Part model, mm, in its own coordinate system. A direction names the side the tool comes from. Round coordinates to 2 decimals unless told otherwise and drop trailing zeros.
from build123d import *

# Parameters (mm, degrees)
SKETCH1_W            = 144.702517086
SKETCH1_H            = 104.868678114
BOSS_EXTRUDE5_DEPTH  = 100
CUT_SWEEP2_PROFILE_R = 5


with BuildPart() as part:
    # Sketch1 → Boss-Extrude5 (new body)
    with BuildSketch(Plane(origin=(0, 0, 0), x_dir=(1, 0, 0), z_dir=(0, 1, 0))):
        Rectangle(SKETCH1_W, SKETCH1_H)
    extrude(amount=BOSS_EXTRUDE5_DEPTH)

    # Cut-Sweep2: sweep along a path in Sketch14
    with BuildLine(Plane(origin=(0, 0, -52.434339057), x_dir=(-1, 0, 0), z_dir=(0, 0, -1))) as cut_sweep2_path:
        Line((-72.351258543, 50), (-29.003803048, 50))
        Line((-29.003803048, 50), (-15.905311349, 69.881639186))
        Line((-15.905311349, 69.881639186), (9.044196649, 69.881639186))
        Line((9.044196649, 69.881639186), (23.390163748, 50))
        Line((23.390163748, 50), (72.351258543, 50))
    # Cut-Sweep2 profile (on start of the path) → Cut-Sweep2 (sweep, cut)
    with BuildSketch(Plane(origin=(72.351258543, 50, -52.434339057), x_dir=(0, 0, -1), z_dir=(-1, 0, 0))):
        Circle(CUT_SWEEP2_PROFILE_R)
    sweep(path=cut_sweep2_path.line, transition=Transition.RIGHT, mode=Mode.SUBTRACT)


solid = part.part
1) Tool access for faces 1 (the face through (3.287, 69.772, -47.436)), 2 (the face through (49.009, 49.89, -47.436)), 3 (the face through (-1, 0, -1)): list every direction of +Z, -Z, +X, -X, +Y, -Y with a clear straight run to the whole face (end or side of a thin tool).
Values:
face 1: -Z
face 2: -Z, +X
face 3: +Z, -Z, +X, -X, -Y
2) Wall check: line 1 along Z through (x, y) = (-10.5, 68.5); line 2 along Z through (x, y) = (56, 46). Give the ranges that are in metal, low to high.
Values:
line 1: z = -47.45 to 52.43
line 2: z = -49.43 to 52.43
3) Drop a flat-ended pin along its axis: pin 1 Ø3 at (x, z) = (-30.5, 12) entering from -Y. Give the stop position or say it passes through.
Values:
pin 1: stops at y = 0
4) Mould opens along X. For faces 4 (the face through (22.25, 60.051, -47.436)), 5 (the face through (72.351, 49, 1)), 6 (the face through (-46.952, 49.89, -47.436)) say: released by +X, released by -X, zero draft, split by the parting line, or undercut.
Values:
face 4: undercut
face 5: released by +X
face 6: zero draft
